```python
from build123d import *

# Parameters (mm, degrees)
SKETCH1_W           = 66.43745389
SKETCH1_H           = 39.85
BOSS_EXTRUDE1_DEPTH = 20
SKETCH2_W           = 30.48
SKETCH2_H           = 39.85
CUT_EXTRUDE1_DEPTH  = 15.02
SKETCH3_W           = 66.43745389
SKETCH3_H           = 39.85
CUT_EXTRUDE2_DEPTH  = 0.75


with BuildPart() as part:
    # Sketch1 → Boss-Extrude1 (new body)
    with BuildSketch(Plane.XY):
        Rectangle(SKETCH1_W, SKETCH1_H)
    extrude(amount=BOSS_EXTRUDE1_DEPTH)

    # Sketch2 → Cut-Extrude1 (cut)
    with BuildSketch(Plane.XY.offset(20)):
        Rectangle(SKETCH2_W, SKETCH2_H)
    extrude(amount=-CUT_EXTRUDE1_DEPTH, mode=Mode.SUBTRACT)

    # Sketch3 → Cut-Extrude2 (cut)
    with BuildSketch(Plane.XY.offset(20)):
        Rectangle(SKETCH3_W, SKETCH3_H)
    extrude(amount=-CUT_EXTRUDE2_DEPTH, mode=Mode.SUBTRACT)


solid = part.part
```
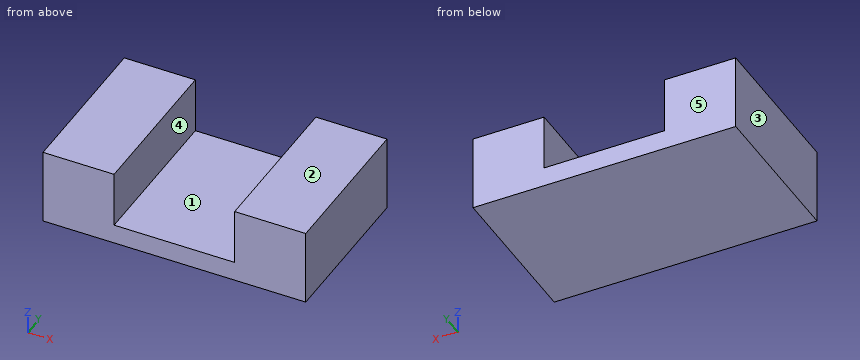
Input: part model. Units: mm. Frame: model coordinates. Face numbers are marked on the shaded views. A direction names the side the tool comes from. Coordinates: 2 decimals unless noted, no trailing zeros. Loops run counter-clockwise (first coordinate to the right, second up) from the corner with the lowest first, then second, coordinate; pieces in that order, holes last. Notation, with made-up numbers: M -31.5,-25 L 3.5,-25 A9 ccw 3.5,-13 Z; hole C 73,58 d11. An arc over 180 degrees is marked long. One line per item, written item: value.
(1) Pull-direction query (X, two-part tool) for the marked faces 1, 2 and 3; classes: +X half, -X half, draft (parallel to the pull), parting line (faces both ways), or undercut.
Filled in:
face 1: undercut
face 2: draft
face 3: -X half
(2) Reachability of the marked faces 4 and 5 from +Z, -Z, +X, -X, +Y, -Y: full face, straight path, thin tool, end or side. Return the list, or none.
Filled in:
face 4: +Z, +Y, -Y
face 5: +Z, -Z, +X, -X, +Y
(3) Section A-A (z = 12.75). Output: boundary loops of the cut face in (x, y) (3 decimals).
Filled in:
outline: M -33.219,-19.925 L -15.24,-19.925 L -15.24,19.925 L -33.219,19.925 Z; M 15.24,-19.925 L 33.219,-19.925 L 33.219,19.925 L 15.24,19.925 Z
(4) Section C-C (x = -3.5). Output: boundary loops of the cut face in (y, z) (3 decimals), and give its area (3 significant figures).
Filled in:
outline: M -19.925,0 L 19.925,0 L 19.925,4.98 L -19.925,4.98 Z
area: 198 mm^2
(5) Line query: line 1 along X through (y, z) = (12, 9.25); line 2 along Z through (x, y) = (0.5, -11). Output: solid intervals per line, ascending. Write a range as from..to.
Filled in:
line 1: -33.22..-15.24, 15.24..33.22
line 2: 0..4.98
(6) Section B-B (y = 15.5). Output: boundary loops of the cut face in (x, z).
Filled in:
outline: M -33.22,0 L 33.22,0 L 33.22,19.25 L 15.24,19.25 L 15.24,4.98 L -15.24,4.98 L -15.24,19.25 L -33.22,19.25 Z
